Work out the finished part from the listing and answer in its coordinate system (mm). Face numbers are marked on the shaded views. Coordinates: 2 decimals unless noted, no trailing zeros. Order: outer loops, then holes, each group sorted by start corner. A loop starts at its lowest first (then second) coordinate and runs counter-clockwise, first axis right, second up.
1. Determine the mould class of the marked faces 1, 2 and 3 for opening direction Z: +Z half, -Z half, draft (parallel to the pull), parting line (faces both ways), or undercut.
2. The part is cut by section A-A, the plane y = 9. Give the vertices of the cut face in (x, z), then the cut area to 3 significant figures.
3. The part is cut by section B-B, the plane y = 4.25. Give the vertices of the cut face in (x, z).
4. Find the intervals of material crossed by probe 1 along Y at (x, z) = (-3, 12.5); probe 2 along Z at (x, y) = (1.5, 8); probe 3 along X at (y, z) = (8.25, 6.75), in increasing order.
5. Flat-ended cylindrical pins translate along their axes: pin 1 Ø2.5 at (x, y) = (-1.5, 9) entering from -Z; pin 2 Ø4 at (x, z) = (-3.5, 3.5) entering from +Y; pin 3 Ø1 at (x, y) = (-9.5, 7.5) entering from +Z. Find the tip coordinate at first contact, or state that the pin passes through.
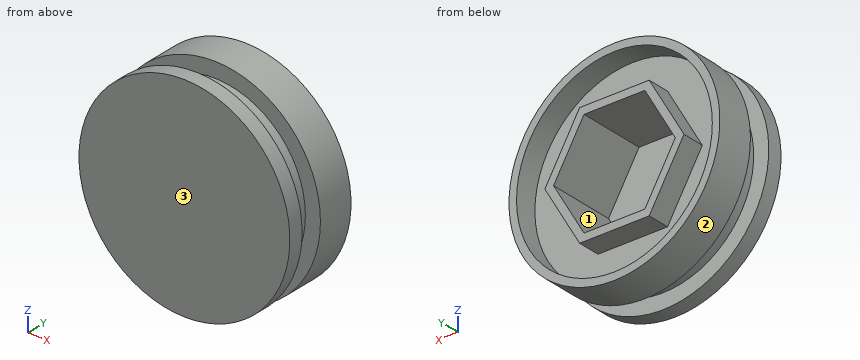
```python
from build123d import *

# Parameters (mm, degrees)
SKETCH1_R           = 14
BOSS_EXTRUDE1_DEPTH = 10
SKETCH2_R           = 13
CUT_EXTRUDE1_DEPTH  = 3
BOSS_EXTRUDE2_DEPTH = 3
CUT_EXTRUDE2_DEPTH  = 9
SKETCH5_W           = 2
SKETCH5_H           = 3


with BuildPart() as part:
    # Sketch1 → Boss-Extrude1 (new body)
    with BuildSketch(Plane(origin=(0, 0, 0), x_dir=(1, 0, 0), z_dir=(0, 1, 0))):
        with Locations(Location((0, 0, 0), (0, 0, 270))):
            Circle(SKETCH1_R)
    extrude(amount=BOSS_EXTRUDE1_DEPTH)

    # Sketch2 → Cut-Extrude1 (cut)
    with BuildSketch(Plane(origin=(0, 10, 0), x_dir=(1, 0, 0), z_dir=(0, 1, 0))):
        with Locations(Location((0, 0, 0), (0, 0, 270))):
            Circle(SKETCH2_R)
    extrude(amount=-CUT_EXTRUDE1_DEPTH, mode=Mode.SUBTRACT)

    # Sketch3 → Boss-Extrude2 (add)
    with BuildSketch(Plane(origin=(0, 7, 0), x_dir=(1, 0, 0), z_dir=(0, 1, 0))):
        Polygon((9.237604307, 0), (4.618802154, 8), (-4.618802154, 8), (-9.237604307, 0), (-4.618802154, -8), (4.618802154, -8), align=None)
    extrude(amount=BOSS_EXTRUDE2_DEPTH)

    # Sketch4 → Cut-Extrude2 (cut)
    with BuildSketch(Plane(origin=(0, 10, 0), x_dir=(1, 0, 0), z_dir=(0, 1, 0))):
        Polygon((8.082903769, 0), (4.041451884, 7), (-4.041451884, 7), (-8.082903769, 0), (-4.041451884, -7), (4.041451884, -7), align=None)
    extrude(amount=-CUT_EXTRUDE2_DEPTH, mode=Mode.SUBTRACT)

    # Cut-Sweep1: sweep along a path in Sketch6
    with BuildLine(Plane(origin=(0, 3.5, 0), x_dir=(1, 0, 0), z_dir=(0, 1, 0))) as cut_sweep1_path:
        CenterArc((0, 0), 13, 0, 360)
    # Sketch5 → Cut-Sweep1 (sweep, cut)
    with BuildSketch(Plane.XY):
        with Locations((13, 3.5)):
            Rectangle(SKETCH5_W, SKETCH5_H)
    sweep(path=cut_sweep1_path.line, mode=Mode.SUBTRACT)


solid = part.part
```
Geometry says:
1. face 1: undercut
1. face 2: parting line
1. face 3: draft
2. outline: circle Ø28 at (0, 0); (-9.24, 0) - (-4.62, -8) - (4.62, -8) - (9.24, 0) - (4.62, 8) - (-4.62, 8) - close; hole circle Ø26 at (0, 0); hole (-8.08, 0) - (-4.04, -7) - (4.04, -7) - (8.08, 0) - (4.04, 7) - (-4.04, 7) - close
2. area: 137 mm2
3. outline: circle Ø24 at (0, 0); hole (-8.08, 0) - (-4.04, -7) - (4.04, -7) - (8.08, 0) - (4.04, 7) - (-4.04, 7) - close
4. probe 1: y = 0 to 2, 5 to 7
4. probe 2: z = -13.92 to -12.91, -8 to -7, 7 to 8, 12.91 to 13.92
4. probe 3: x = -12.27 to -11.11, -5.34 to -4.19, 4.19 to 5.34, 11.11 to 12.27
5. pin 1: stops at z = -14
5. pin 2: stops at y = 1
5. pin 3: stops at z = 10.72
